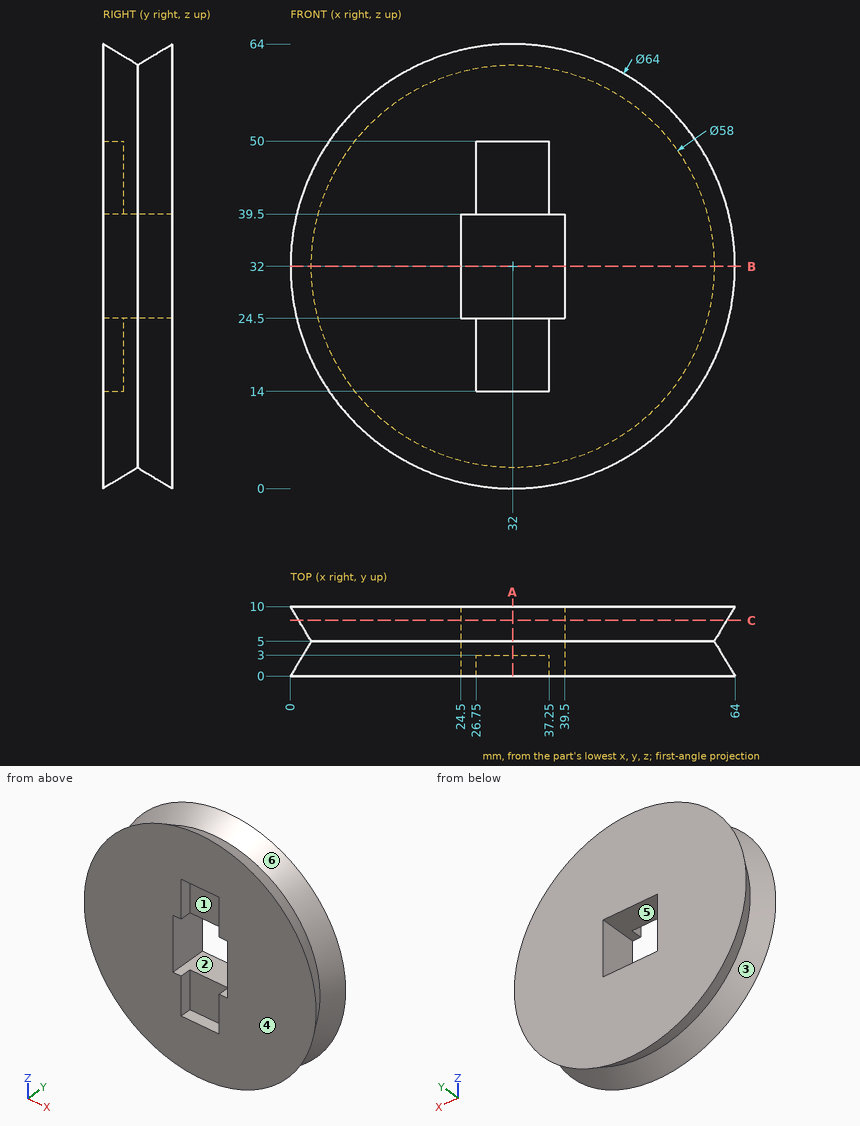
Geometry: see drawing. Coordinates: mm, zero at the bounding-box minimum. A direction names the side the tool comes from. Coordinates: 2 decimals unless noted, no trailing zeros. Loops run counter-clockwise (first coordinate to the right, second up) from the corner with the lowest first, then second, coordinate; pieces in that order, holes last.
(1) Section C-C on y = 8. Return the cut outline in (x, z), then the cut area to 3 significant figures.
(2) Pull-direction query (X, two-part tool) for the marked faces 4, 5 and 6; classes: released by +X, released by -X, zero draft, split by the parting line, or undercut.
(3) Set-up query: the marked faces 1, 2 and 3. Return all of +Z, -Z, +X, -X, +Y, -Y with unobstructed straight access to the full face (end or side cutting, diameter ignored); none if empty.
(4) Section A-A on x = 32. Return the cut outline in (y, z).
(5) Material intervals for probe 1 along Y at (x, z) = (57, 50.5); probe 2 along X at (y, z) = (2.5, 29.5); probe 3 along X at (y, z) = (3.75, 26), sorted ascending.
(6) Section B-B on z = 32. Return the cut outline in (x, y).
(7) First-contact query: pin 1 Ø2.5 at (y, z) = (2, 43) entering from +X; pin 2 Ø1.5 at (y, z) = (1.5, 20.5) entering from -X; pin 3 Ø2.5 at (x, y) = (32.5, 2) entering from -Z; pin 4 Ø12 at (x, z) = (27.5, 27.5) entering from -Y. Flat tips, straight axial feed; report the tip coordinate or a pass-through.
Data:
1. outline: circle Ø61.6 at (32, 32); hole (24.5, 24.5) - (39.5, 24.5) - (39.5, 39.5) - (24.5, 39.5) - close
1. area: 2,760 mm2
2. face 4: zero draft
2. face 5: undercut
2. face 6: split by the parting line
3. face 1: -Y
3. face 2: +Y, -Y
3. face 3: none
4. outline: (0, 0) - (5, 3) - (10, 0) - (10, 24.5) - (3, 24.5) - (3, 14) - (0, 14) - close; (0, 50) - (3, 50) - (3, 39.5) - (10, 39.5) - (10, 64) - (5, 61) - (0, 64) - close
5. probe 1: y = 0 to 1.5, 8.5 to 10
5. probe 2: x = 1.6 to 24.5, 39.5 to 62.4
5. probe 3: x = 2.86 to 24.5, 39.5 to 61.14
6. outline: (0, 0) - (24.5, 0) - (24.5, 10) - (0, 10) - (3, 5) - close; (39.5, 0) - (64, 0) - (61, 5) - (64, 10) - (39.5, 10) - close
7. pin 1: stops at x = 61.69
7. pin 2: stops at x = 2.54
7. pin 3: stops at z = 0.45
7. pin 4: stops at y = 0
